Geometry check sheet. Reference: the model listing, model coordinates, mm. Face numbers are marked on the shaded views. A direction names the side the tool comes from. Give positions to 0.01 mm unless a question says otherwise; leave off trailing zeros. Loops run counter-clockwise (first coordinate to the right, second up) from the corner with the lowest first, then second, coordinate; pieces in that order, holes last. Notation, with made-up numbers: (-15.75, 60) -> (30.25, 60) arc R22 cw to (30.25, 87) -> close; hole circle Ø11 at (35.25, 21.25). An arc over 180 degrees is marked (long way). Write item = value, one per line.
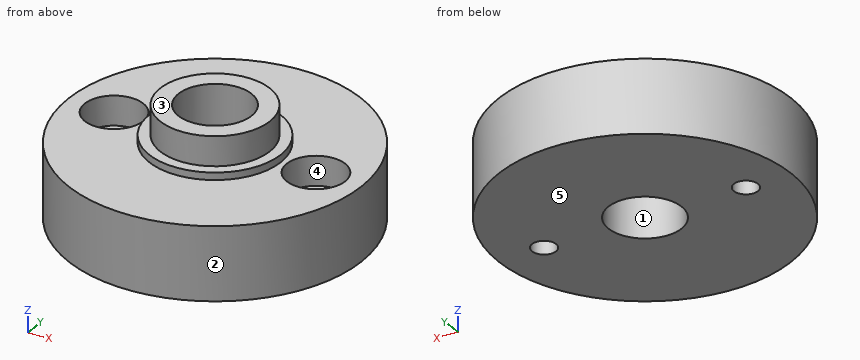
```python
from build123d import *

# Parameters (mm, degrees)
SKETCH_1_R          = 20
SKETCH_1_R_2        = 5
SKETCH_1_R_3        = 1.65
EXTRUDE_1_DEPTH     = 10
SKETCH_2_R          = 9
SKETCH_2_R_2        = 5
EXTRUDE_2_DEPTH     = 1
SKETCH_3_R          = 7.5
SKETCH_3_R_2        = 5
EXTRUDE_3_DEPTH     = 4
SKETCH_4_R          = 4
CUT_EXTRUDE_1_DEPTH = 4


with BuildPart() as part:
    # ｽｹｯﾁ1 → ﾎﾞｽ - 押し出し1 (new body)
    with BuildSketch(Plane.XY):
        Circle(SKETCH_1_R)
        Circle(SKETCH_1_R_2, mode=Mode.SUBTRACT)
        with Locations((-13.75, 0)):
            Circle(SKETCH_1_R_3, mode=Mode.SUBTRACT)
        with Locations((13.75, 0)):
            Circle(SKETCH_1_R_3, mode=Mode.SUBTRACT)
    extrude(amount=EXTRUDE_1_DEPTH)

    # ｽｹｯﾁ2 → ﾎﾞｽ - 押し出し2 (add)
    with BuildSketch(Plane.XY.offset(10)):
        Circle(SKETCH_2_R)
        Circle(SKETCH_2_R_2, mode=Mode.SUBTRACT)
    extrude(amount=EXTRUDE_2_DEPTH)

    # ｽｹｯﾁ3 → ﾎﾞｽ - 押し出し3 (add)
    with BuildSketch(Plane.XY.offset(11)):
        Circle(SKETCH_3_R)
        Circle(SKETCH_3_R_2, mode=Mode.SUBTRACT)
    extrude(amount=EXTRUDE_3_DEPTH)

    # ｽｹｯﾁ4 → ｶｯﾄ - 押し出し1 (cut)
    with BuildSketch(Plane.XY.offset(10)):
        with Locations((-13.75, 0)):
            Circle(SKETCH_4_R)
        with Locations((13.75, 0)):
            Circle(SKETCH_4_R)
    extrude(amount=-CUT_EXTRUDE_1_DEPTH, mode=Mode.SUBTRACT)


solid = part.part
```
Item 1: Section check B-B, the plane y = 0. Give the number of separate pieces and of enclosed holes in the cut face, plus the area to 3 significant figures.
Answer:
separate_pieces = 4
enclosed_holes = 0
area = 224 mm^2
Item 2: Section check A-A, the plane x = 13.75. Record the cut outline in (y, z).
Answer:
outline = (-14.52, 0) -> (-1.65, 0) -> (-1.65, 6) -> (-4, 6) -> (-4, 10) -> (-14.52, 10) -> close; (1.65, 0) -> (14.52, 0) -> (14.52, 10) -> (4, 10) -> (4, 6) -> (1.65, 6) -> close
Item 3: Section check D-D, the plane x = -14. Record the cut outline in (y, z).
Answer:
outline = (-14.28, 0) -> (-1.63, 0) -> (-1.63, 6) -> (-3.99, 6) -> (-3.99, 10) -> (-14.28, 10) -> close; (1.63, 0) -> (14.28, 0) -> (14.28, 10) -> (3.99, 10) -> (3.99, 6) -> (1.63, 6) -> close
Item 4: Section check C-C, the plane z = 6.5. Record the cut outline in (x, y).
Answer:
outline = circle Ø40 at (0, 0); hole circle Ø8 at (-13.75, 0); hole circle Ø10 at (0, 0); hole circle Ø8 at (13.75, 0)
Item 5: Gauge pin test, flat ends, axial feed: pin 1 (6 mm diameter, centred on x = 8, y = 10.5, fed in from +Z); pin 2 (1 mm diameter, centred on x = 2, z = 3.5, fed in from +Y); pin 3 (6.5 mm diameter, centred on x = -13.75, y = 0, fed in from +Z). Record the tip position at first contact, or that the pin passes through.
Answer:
pin_1 = 10
pin_2 = 19.94
pin_3 = 6
Item 6: Thickness scan on L1, parallel to Y at x = 0, z = 3.75; L2, parallel to Z at x = 12.5, y = -14.5; L3, parallel to Y at x = 13.75, z = 2.15. Record the ranges inside material, lowest first. Write a range as [from, to].
Answer:
L1 = [-20, -5], [5, 20]
L2 = [0, 10]
L3 = [-14.52, -1.65], [1.65, 14.52]
Item 7: Tool access check on the marked faces 4 and 5. Record the directions out of +Z, -Z, +X, -X, +Y, -Y that give a thin tool (end or side, any length) a straight path to the whole face; none if there is none.
Answer:
face_4 = +Z
face_5 = -Z, +X, -X, +Y, -Y
Item 8: Draft check along X on the marked faces 1, 2 and 3. Enter one of: +X half, -X half, draft (parallel to the pull), parting line (faces both ways), or undercut.
Answer:
face_1 = undercut
face_2 = parting line
face_3 = draft
